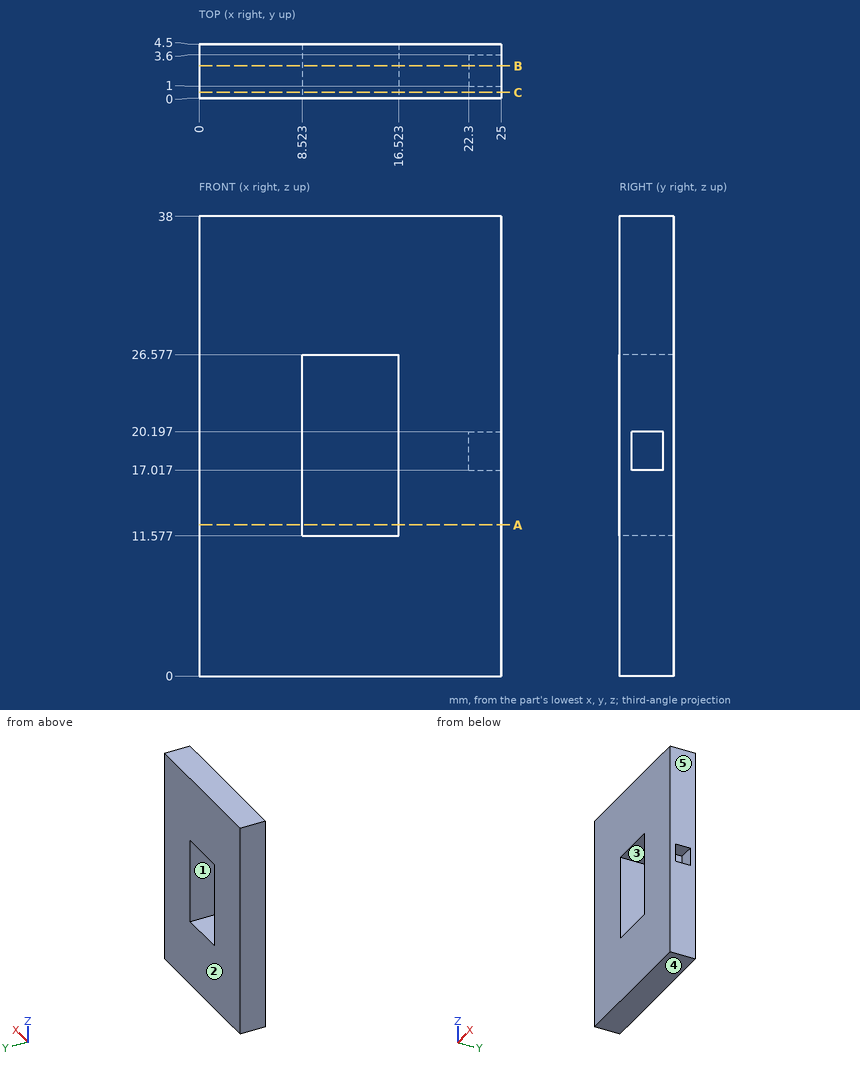
Design review of the part shown in the three views and the two pictorial views. Dimensions are in mm from the part's minimum x, y and z. A direction names the side the tool comes from. Give positions to 0.01 mm unless a question says otherwise; leave off trailing zeros. Loops run counter-clockwise (first coordinate to the right, second up) from the corner with the lowest first, then second, coordinate; pieces in that order, holes last. Notation, with made-up numbers: (51, 43) -> (76, 43) arc R25 cw to (76, 77) -> close; hole circle Ø5 at (-24.5, -31). An arc over 180 degrees is marked (long way). One line per item, written item: value.
Q1. For pin 1 Ø0.8 at (y, z) = (2, 19) entering from +X, flat-tipped, find the tip position at first contact; note if it passes through.
Numbers:
pin 1: stops at x = 22.3
Q2. We need section A-A on z = 12.5. Give the boundary of the cut face in (x, y), and give its area (3 significant figures).
Numbers:
outline: (0, 0) -> (8.52, 0) -> (8.52, 4.5) -> (0, 4.5) -> close; (16.52, 0) -> (25, 0) -> (25, 4.5) -> (16.52, 4.5) -> close
area: 76.5 mm^2
Q3. Machinability: for the marked faces 1 and 2, which of the approach directions +Z, -Z, +X, -X, +Y, -Y give a long, thin tool a straight path to every point of the face, cutting with its end or side? Answer none if there is none.
Numbers:
face 1: +Y, -Y
face 2: +Z, -Z, +X, -X, +Y
Q4. We need section B-B on y = 2.7. Give the boundary of the cut face in (x, z).
Numbers:
outline: (0, 0) -> (25, 0) -> (25, 17.02) -> (22.3, 17.02) -> (22.3, 20.2) -> (25, 20.2) -> (25, 38) -> (0, 38) -> close; hole (8.52, 11.58) -> (16.52, 11.58) -> (16.52, 26.58) -> (8.52, 26.58) -> close
Q5. Draft analysis for pull direction X (two halves, no side actions). For the marked faces 3, 4 and 5, state which applies: pulls with the +X half, pulls with the -X half, needs draft (parallel to the pull), parting line crosses it, or undercut.
Numbers:
face 3: undercut
face 4: needs draft
face 5: pulls with the +X half
Q6. We need section C-C on y = 0.5. Give the boundary of the cut face in (x, z), and give its area (3 significant figures).
Numbers:
outline: (0, 0) -> (25, 0) -> (25, 38) -> (0, 38) -> close; hole (8.52, 11.58) -> (16.52, 11.58) -> (16.52, 26.58) -> (8.52, 26.58) -> close
area: 830 mm^2
Q7. For L1, parallel to X at y = 3.95, z = 21; L2, parallel to Z at x = 13.25, y = 3.5, list the stretches that pass through material, from the lowest coordinate up.
Numbers:
L1: x = 0 to 8.52, 16.52 to 25
L2: z = 0 to 11.58, 26.58 to 38
